```python
from build123d import *

# Parameters (mm, degrees)
F0_W     = 600
F0_H     = 450
F1_DEPTH = 16
F2_W     = 150
F2_H     = 120
F3_DEPTH = 16.001
F4_R     = 10


with BuildPart() as f1:
    # F0 (on Top) → F1 (new body)
    with BuildSketch(Plane.XY):
        Rectangle(F0_W, F0_H)
    extrude(amount=F1_DEPTH)

    # F2 (on face) → F3 (cut, through all)
    with BuildSketch(Plane.XY.offset(16)):
        Rectangle(F2_W, F2_H)
    extrude(amount=-F3_DEPTH, mode=Mode.SUBTRACT)

    # F4
    f4_edges = [f1.edges().sort_by_distance(p)[0] for p in [
        (-75, 60, 8),
        (75, 60, 8),
        (75, -60, 8),
        (-75, -60, 8),
    ]]
    fillet(f4_edges, radius=F4_R)


solid = f1.part
```
Source: CAD feature listing. Evaluate the final solid. Frame: model axes, mm. A direction names the side the tool comes from. Round coordinates to 2 decimals unless told otherwise and drop trailing zeros. Loops run counter-clockwise (first coordinate to the right, second up) from the corner with the lowest first, then second, coordinate; pieces in that order, holes last. Notation, with made-up numbers: M 1.25,4 L 6.25,4 A13 cw 6.25,10 Z; hole C 51.25,64 d11. An arc over 180 degrees is marked long. Use a Markdown table: item, result. Add a question column.
1. Cut plane C-C, the plane x = -56.5. Output: boundary loops of the cut face in (y, z).
2. Contact query for a flat-ended pin moving along its axis: pin 1 (8 mm diameter, centred on x = 108.5, y = 124, fed in from -Z). Output: stop coordinate, or through.
3. Cut plane B-B, the plane z = 4. Output: boundary loops of the cut face in (x, y).
4. Set-up query: faces 1 (the flat face through (-4, 103, 0)), 2 (the flat face through (75, -1, 8)). Return all of +Z, -Z, +X, -X, +Y, -Y with unobstructed straight access to the full face (end or side cutting, diameter ignored); none if empty.
5. Ray query, line 1 along X through (y, z) = (40, 5); line 2 along Y through (x, z) = (25, 4.25). Return the intervals inside material, ascending. Write a range as [from, to].
6. Cut plane A-A, the plane y = -15. Output: boundary loops of the cut face in (x, z), and give its area (3 significant figures).
7. Pull-direction query (Y, two-part tool) for faces 3 (the flat face through (-1, -60, 8)), 4 (the flat face through (-4, 225, 8)), 5 (the flat face through (-300, -3, 8)); classes: +Y half, -Y half, draft (parallel to the pull), parting line (faces both ways), or undercut.
Solution:
| question | item | result |
|---|---|---|
| 1 | outline | M -225,0 L -60,0 L -60,16 L -225,16 Z; M 60,0 L 225,0 L 225,16 L 60,16 Z |
| 2 | pin 1 | stops at z = 0 |
| 3 | outline | M -300,-225 L 300,-225 L 300,225 L -300,225 Z; hole M -75,-50 A10 ccw -65,-60 L 65,-60 A10 ccw 75,-50 L 75,50 A10 ccw 65,60 L -65,60 A10 ccw -75,50 Z |
| 4 | face 1 | -Z, +X, -X, +Y, -Y |
| 4 | face 2 | +Z, -Z |
| 5 | line 1 | x = [-300, -75], [75, 300] |
| 5 | line 2 | y = [-225, -60], [60, 225] |
| 6 | outline | M -300,0 L -75,0 L -75,16 L -300,16 Z; M 75,0 L 300,0 L 300,16 L 75,16 Z |
| 6 | area | 7,200 mm2 |
| 7 | face 3 | undercut |
| 7 | face 4 | +Y half |
| 7 | face 5 | draft |
